from build123d import *

# Parameters (mm, degrees)
F1_DEPTH = 75
F2_R     = 5


with BuildPart() as f1:
    # F0 (on Top) → F1 (new body)
    with BuildSketch(Plane.XY):
        with BuildLine():
            Line((-23.66752, 26.337069), (-23.66752, -18.662931))
            Line((-23.66752, -18.662931), (41.33248, -18.662931))
            Line((41.33248, -18.662931), (41.33248, 26.337069))
            Line((41.33248, 26.337069), (31.841161, 26.337069))
            ThreePointArc((31.841161, 26.337069), (8.445234, 8.710863), (-14.950693, 26.337069))
            Line((-14.950693, 26.337069), (-23.66752, 26.337069))
        make_face()
    extrude(amount=F1_DEPTH)

    # F2
    f2_edges = [f1.edges().sort_by_distance(p)[0] for p in [
        (41.33248, -18.662931, 37.5),
    ]]
    fillet(f2_edges, radius=F2_R)


solid = f1.part
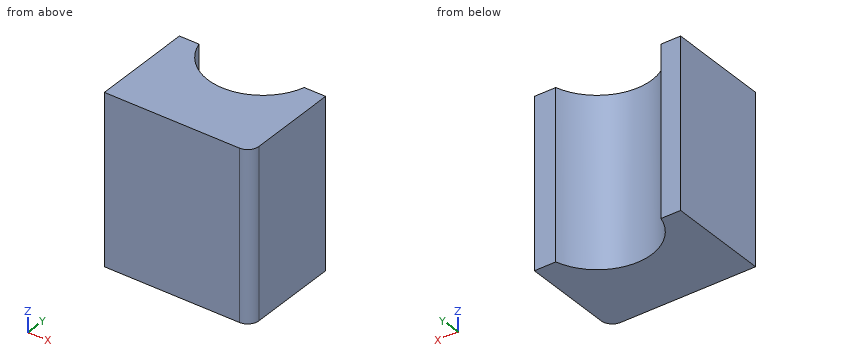
Check sheet for the modelled part. Datum: model origin and axes. Units: mm. Coordinates: 2 decimals unless noted, no trailing zeros. Write each loop counter-clockwise with the first axis right and the second up, starting at its lowest first coordinate (ties: lowest second). Pieces come first, ordered by that corner, then holes.
Item 1: Scan lines: probe 1 along X at (y, z) = (13.5, 46); probe 2 along X at (y, z) = (17.5, 32.5); probe 3 along X at (y, z) = (-14.5, 26.5). Record each from-to range of solid material in increasing order.
Numbers:
probe 1: x = -23.67 to -6.05, 22.94 to 41.33
probe 2: x = -23.67 to -10.28, 27.17 to 41.33
probe 3: x = -23.67 to 41.26
Item 2: Cross-section at B-B on x = 21. Record the boundary of the cut face in (y, z), then the cut area to 3 significant figures.
Numbers:
outline: (-18.66, 0) - (12.2, 0) - (12.2, 75) - (-18.66, 75) - close
area: 2,310 mm2
Item 3: Cross-section at A-A on z = 14. Record the boundary of the cut face in (x, y).
Numbers:
outline: (-23.67, -18.66) - (36.33, -18.66) arc R5 ccw to (41.33, -13.66) - (41.33, 26.34) - (31.84, 26.34) arc R24.34 cw to (-14.95, 26.34) - (-23.67, 26.34) - close
Item 4: Depth check by flat-ended pin: pin 1 Ø8 at (x, z) = (24, 32) entering from +Y. Enter the tip coordinate at first touch or a pass-through.
Numbers:
pin 1: stops at y = 18.56
Item 5: Cross-section at C-C on x = 27.5. Record the boundary of the cut face in (y, z).
Numbers:
outline: (-18.66, 0) - (17.91, 0) - (17.91, 75) - (-18.66, 75) - close
